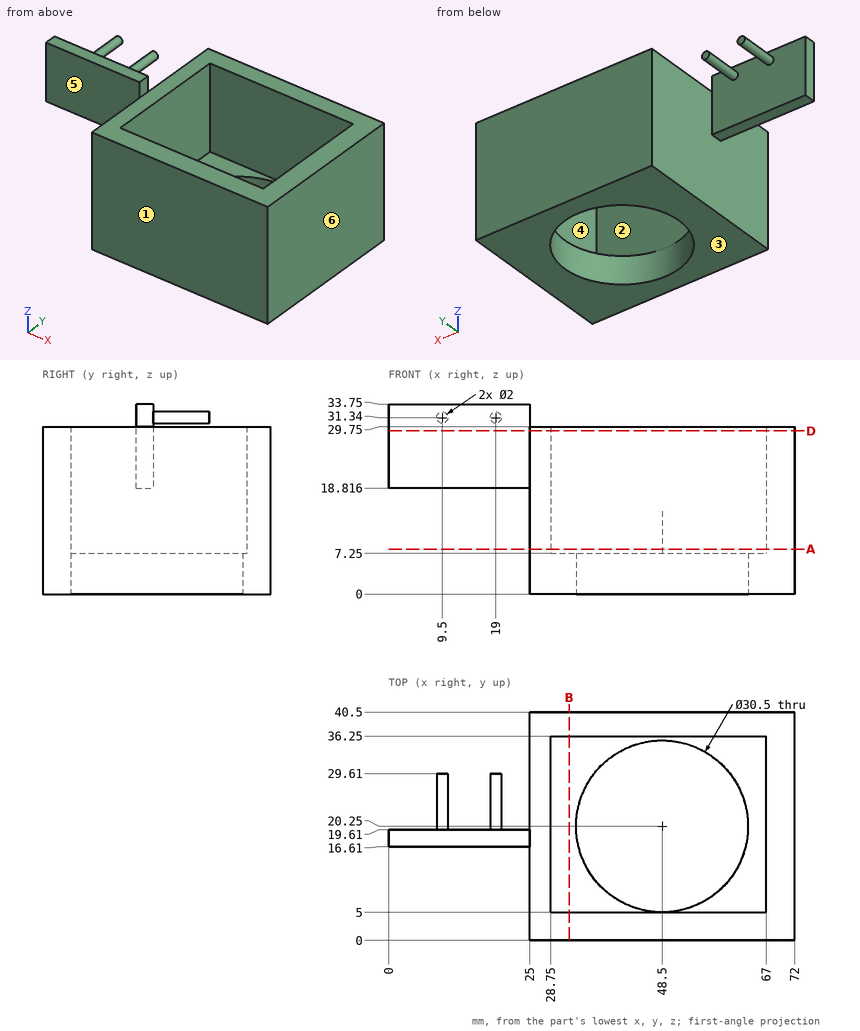
Geometry: see drawing. Coordinates: mm, zero at the bounding-box minimum. A direction names the side the tool comes from. Coordinates: 2 decimals unless noted, no trailing zeros. Loops run counter-clockwise (first coordinate to the right, second up) from the corner with the lowest first, then second, coordinate; pieces in that order, holes last. Notation, with made-up numbers: M 32,31 L 90,31 A32 cw 90,62 Z; hole C -35.75,-20 d10. An arc over 180 degrees is marked long. Answer in a Markdown table with one row per item.
1. Draft query along Y for the marked faces 1, 2 and 3. Return one class per face: pulls with the +Y half, pulls with the -Y half, needs draft (parallel to the pull), parting line crosses it, or undercut.
Response:
| item | result |
|---|---|
| face 1 | pulls with the -Y half |
| face 2 | undercut |
| face 3 | needs draft |
2. Section A-A, the plane z = 8. Output: boundary loops of the cut face in (x, y), then the cut area to 3 significant figures.
Response:
| item | result |
|---|---|
| outline | M 25,0 L 72,0 L 72,40.5 L 25,40.5 Z; hole M 28.75,5 L 67,5 L 67,36.25 L 28.75,36.25 Z |
| area | 708 mm2 |
3. First-contact query: pin 1 (1 mm diameter, centred on y = 30, z = 9.5, fed in from -X); pin 2 (2 mm diameter, centred on x = 9.5, z = 31, fed in from +Y); pin 3 (3.5 mm diameter, centred on x = 18.5, y = 18, fed in from -Z); pin 4 (18 mm diameter, centred on y = 14.5, z = 20.5, fed in from -X). Flat tips, straight axial feed; report the tip coordinate or a pass-through.
Response:
| item | result |
|---|---|
| pin 1 | stops at x = 25 |
| pin 2 | stops at y = 29.61 |
| pin 3 | stops at z = 18.82 |
| pin 4 | stops at x = 0 |
4. Section D-D, the plane z = 29. Output: boundary loops of the cut face in (x, y).
Response:
| item | result |
|---|---|
| outline | M 0,16.61 L 25,16.61 L 25,0 L 72,0 L 72,40.5 L 25,40.5 L 25,19.61 L 0,19.61 Z; hole M 28.75,5 L 67,5 L 67,36.25 L 28.75,36.25 Z |
5. Material intervals for line 1 (Y direction, x = 39.5, z = 21); line 2 (X direction, y = 10, z = 25.5); line 3 (Y direction, x = 48.5, z = 5), sorted ascending.
Response:
| item | result |
|---|---|
| line 1 | y = 0 to 5, 36.25 to 40.5 |
| line 2 | x = 25 to 28.75, 67 to 72 |
| line 3 | y = 0 to 5, 35.5 to 40.5 |
6. Section B-B, the plane x = 32. Output: boundary loops of the cut face in (y, z).
Response:
| item | result |
|---|---|
| outline | M 0,0 L 40.5,0 L 40.5,29.75 L 36.25,29.75 L 36.25,7.25 L 5,7.25 L 5,29.75 L 0,29.75 Z |
7. Reachability of the marked faces 4, 5 and 6 from +Z, -Z, +X, -X, +Y, -Y: full face, straight path, thin tool, end or side. Return the list, or none.
Response:
| item | result |
|---|---|
| face 4 | +Z |
| face 5 | +Z, -Z, -X, -Y |
| face 6 | +Z, -Z, +X, +Y, -Y |
